Design review of the part built by this model. Coordinates are the model's own, in mm. Face numbers are marked on the shaded views. A direction names the side the tool comes from. Give positions to 0.01 mm unless a question says otherwise; leave off trailing zeros. Write each loop counter-clockwise with the first axis right and the second up, starting at its lowest first coordinate (ties: lowest second). Pieces come first, ordered by that corner, then holes.
```python
from build123d import *

# Parameters (mm, degrees)
F1_DEPTH = 63.5
F0_W     = 25.4
F0_H     = 19.05
F2_DEPTH = 25.4
F3_DEPTH = 7.9375
F5_R     = 6.35
F6_R     = 6.35


# Not quite as in the source:
# - a feature names something its author has since deleted; it is built from what else it names


with BuildPart() as f1:
    # F0 (on Front) → F1 (new body, symmetric)
    with BuildSketch(Plane.XZ):
        Polygon((22.225, 9.525), (-41.275, 9.525), (-41.275, -9.525), (41.275, -9.525), (41.275, 9.525), align=None)
    extrude(amount=F1_DEPTH, both=True)

    # F0 (on Front) → F2 (join, symmetric)
    with BuildSketch(Plane.XZ):
        with BuildLine():
            Line((22.225, 27.0002), (22.225, 9.525))
            Line((22.225, 9.525), (41.275, 9.525))
            Line((41.275, 9.525), (41.275, 27.0002))
            ThreePointArc((41.275, 27.0002), (45.9246798487, 38.2255201513), (57.15, 42.8752))
            Line((57.15, 42.8752), (60.325, 42.8752))
            Line((60.325, 42.8752), (60.325, 61.9252))
            Line((60.325, 61.9252), (57.15, 61.9252))
            add(Edge.make_bspline(
                [(55.6286861057, 61.8920504673), (56.1384142752, 61.9045266367), (56.6455676592, 61.915561496), (57.15, 61.9252)],
                knots=[110.1136190258, 110.1136190258, 110.1136190258, 110.1136190258, 111.5045361635, 111.5045361635, 111.5045361635, 111.5045361635], degree=3))
            ThreePointArc((55.6286861057, 61.8920504673), (31.9221630658, 51.1520502111), (22.225, 27.0002))
        make_face()
        with Locations((73.025, 52.4002)):
            Rectangle(F0_W, F0_H)
    extrude(amount=F2_DEPTH, both=True)

    # F0 (on Front) → F3 (join, symmetric)
    with BuildSketch(Plane.XZ):
        with BuildLine():
            add(Edge.make_bspline(
                [(-41.275, 9.525), (-41.2147135228, 50.8835652719), (15.2754458257, 60.9043595954), (55.6286861057, 61.8920504673)],
                knots=[0, 0, 0, 0, 110.1136190258, 110.1136190258, 110.1136190258, 110.1136190258], degree=3))
            Line((-41.275, 9.525), (22.225, 9.525))
            Line((22.225, 9.525), (22.225, 27.0002))
            ThreePointArc((22.225, 27.0002), (31.9221630658, 51.1520502111), (55.6286861057, 61.8920504673))
        make_face()
    extrude(amount=F3_DEPTH, both=True)

    # F0 (on Front) → F4 (revolve)
    with BuildSketch(Plane.XZ):
        Polygon((85.725, 66.675), (85.725, 61.9252), (85.725, 42.8752), (85.725, 38.1), (111.125, 38.1), (111.125, 66.675), align=None)
    revolve(axis=Axis((85.725, 0, 52.4002), (0, 0, 1)))

    # F5
    f5_edges = [f1.edges().sort_by_distance(p)[0] for p in [
        (-41.275, 63.5, 0),
    ]]
    fillet(f5_edges, radius=F5_R)

    # F6
    f6_edges = [f1.edges().sort_by_distance(p)[0] for p in [
        (-41.275, -63.5, 0),
        (41.275, 63.5, 0),
        (41.275, -63.5, 0),
    ]]
    fillet(f6_edges, radius=F6_R)


solid = f1.part
```
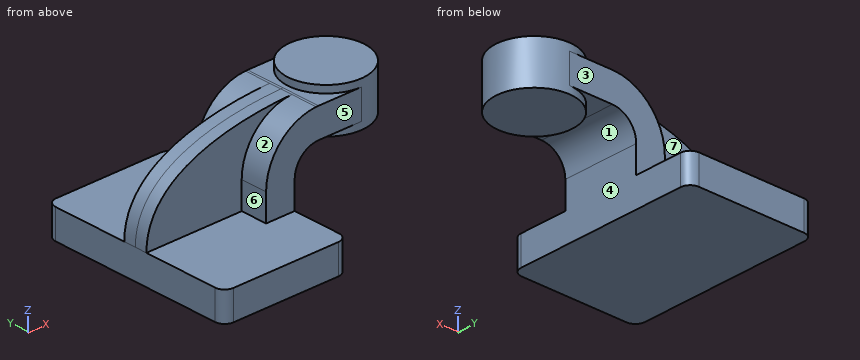
(1) Mouldability with a two-part tool opening along X and no side actions: class the marked faces 1, 2, 3 and 4 as pulls with the +X half, pulls with the -X half, needs draft (parallel to the pull), parting line crosses it, or undercut.
Resolved:
face 1: undercut
face 2: pulls with the -X half
face 3: needs draft
face 4: pulls with the +X half
(2) Consider section D-D, the plane x = 83. Give the boundary of the cut face in (y, z) (3 decimals).
Resolved:
outline: (-25.4, 42.875) - (-25.253, 42.875) - (-25.253, 38.1) - (25.253, 38.1) - (25.253, 42.875) - (25.4, 42.875) - (25.4, 61.925) - (25.253, 61.925) - (25.253, 66.675) - (-25.253, 66.675) - (-25.253, 61.925) - (-25.4, 61.925) - close
(3) To check wall thickness, follow L1, parallel to Y at x = 6, z = 19; L2, parallel to Y at x = -35, z = 1; L3, parallel to X at y = -11, z = 9 (3 decimals). State the ranges of each line that lie inside material, in increasing order.
Resolved:
L1: y = -7.94 to 7.94
L2: y = -63.5 to 63.5
L3: x = -41.275 to 41.275
(4) Clearance check with flat-ended pins moving along their axes: P1, Ø14.5, axis at x = 74.5, y = 1.5, coming from the -Z side; P2, Ø5, axis at y = -17.5, z = 14.5, coming from the -X side (3 decimals); P3, Ø15.5, axis at x = 20.5, z = 45, coming from the -Y side; P4, Ø2, axis at x = 44, z = 24.5, coming from the -Y side. State where each tip first meets the part, or that it passes through.
Resolved:
P1: stops at z = 38.1
P2: stops at x = 22.225
P3: stops at y = -25.4
P4: passes through
(5) Consider section C-C, the plane x = 63. Give the boundary of the cut face in (y, z) (3 decimals).
Resolved:
outline: (-25.4, 42.875) - (-11.346, 42.875) - (-11.346, 38.1) - (11.346, 38.1) - (11.346, 42.875) - (25.4, 42.875) - (25.4, 61.925) - (11.346, 61.925) - (11.346, 66.675) - (-11.346, 66.675) - (-11.346, 61.925) - (-25.4, 61.925) - close
(6) Consider section A-A, the plane z = 6. Give the boundary of the cut face in (x, y) (3 decimals), then the cut area to 3 significant figures.
Resolved:
outline: (-41.275, -57.15) arc R6.35 ccw to (-34.925, -63.5) - (34.925, -63.5) arc R6.35 ccw to (41.275, -57.15) - (41.275, 57.15) arc R6.35 ccw to (34.925, 63.5) - (-34.925, 63.5) arc R6.35 ccw to (-41.275, 57.15) - close
area: 10,400 mm2
(7) Consider section B-B, the plane y = -55. Give the boundary of the cut face in (x, z) (3 decimals), then the cut area to 3 significant figures.
Resolved:
outline: (-41.275, -9.525) - (41.275, -9.525) - (41.275, 9.525) - (-41.275, 9.525) - close
area: 1,570 mm2
(8) Tool access review of the marked faces 5, 6 and 7: name each direction out of +Z, -Z, +X, -X, +Y, -Y from which nothing blocks a thin tool from reaching the whole face with its end or side.
Resolved:
face 5: +Z, +X, -X, -Y
face 6: +Z, -X, -Y
face 7: +Z, -X, +Y
